The model under review builds one solid part; all positions refer to its coordinate system, in mm. Face numbers are marked on the shaded views. A direction names the side the tool comes from. Coordinates: 2 decimals unless noted, no trailing zeros. Order: outer loops, then holes, each group sorted by start corner. A loop starts at its lowest first (then second) coordinate and runs counter-clockwise, first axis right, second up. Notation, with made-up numbers: M 19.5,-10 L 54.5,-10 A18 ccw 54.5,-2 Z; hole C -4,1.25 d7. An arc over 180 degrees is marked long. Answer in a Markdown table with one row per item.
from build123d import *

# Parameters (mm, degrees)
CHAMFER_1_SIZE      = 1.1015
SKETCH_2_W          = 50
SKETCH_2_H          = 3
CUT_EXTRUDE_1_DEPTH = 3.892099643


with BuildPart() as part:
    # Эскиз1 → Повернуть1 (revolve)
    with BuildSketch(Plane.XY):
        with BuildLine():
            Line((0, 12), (5, 12))
            ThreePointArc((5, 12), (8.36795896, 7.179530606), (9.892099643, 1.5))
            Line((9.892099643, 1.5), (7, 1.5))
            Line((7, 1.5), (7, 0))
            Line((7, 0), (3.5, 0))
            Line((3.5, 0), (3.5, 7.5))
            Line((3.5, 7.5), (0, 7.5))
            Line((0, 7.5), (0, 12))
        make_face()
    revolve(axis=Axis((0, 0, 0), (1, 0, 0)))

    # Фаска1
    chamfer_1_edges = [part.edges().sort_by_distance(p)[0] for p in [
        (0, -12, 0),
    ]]
    chamfer(chamfer_1_edges, length=CHAMFER_1_SIZE)

    # Эскиз2 → Вырез-Вытянуть1 (cut, through all)
    with BuildSketch(Plane(origin=(7, 0, 0), x_dir=(0, 0, -1), z_dir=(1, 0, 0))):
        Rectangle(SKETCH_2_W, SKETCH_2_H)
    extrude(amount=CUT_EXTRUDE_1_DEPTH, mode=Mode.SUBTRACT)


solid = part.part
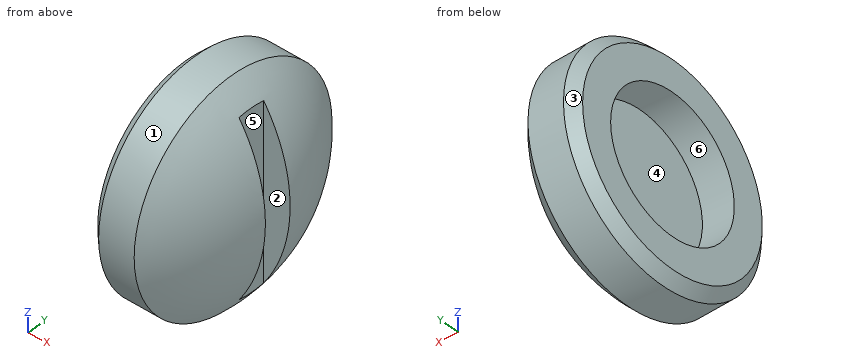
(1) Take a section at A-A (y = 0). Write out the cut boundary in (x, z), then the cut area to 3 significant figures.
Report:
| item | result |
|---|---|
| outline | M 0,-10.9 L 1.1,-12 L 5,-12 A17 ccw 7,-9.58 L 7,9.58 A17 ccw 5,12 L 1.1,12 L 0,10.9 L 0,7.5 L 3.5,7.5 L 3.5,-7.5 L 0,-7.5 Z |
| area | 110 mm^2 |
(2) The part is to be moulded in two halves that separate along Z. For the marked faces 3, 4, 5 and 6, say which applies: +Z half, -Z half, draft (parallel to the pull), parting line (faces both ways), or undercut.
Report:
| item | result |
|---|---|
| face 3 | parting line |
| face 4 | undercut |
| face 5 | draft |
| face 6 | undercut |
(3) Insertion check: P1, Ø3.5, axis at y = 0, z = -3, coming from the +X side; P2, Ø1, axis at x = 4.5, y = -7.5, coming from the -Z side; P3, Ø12, axis at y = 0, z = -0.5, coming from the -X side. Each pin has a flat end and moves straight along its axis. Give the tip position at first contact, or say it passes through.
Report:
| item | result |
|---|---|
| P1 | x = 9.76 |
| P2 | z = -9.75 |
| P3 | x = 3.5 |
(4) Take a section at B-B (x = 2). Write out the cut boundary in (y, z).
Report:
| item | result |
|---|---|
| outline | C 0,0 d24; hole C 0,0 d15 |
(5) Take a section at C-C (x = 5.75). Write out the cut boundary in (y, z), then the cut area to 3 significant figures.
Report:
| item | result |
|---|---|
| outline | C 0,0 d22.39 |
| area | 394 mm^2 |
(6) To check wall thickness, follow line 1 (Z direction, x = 1.55, y = 0); line 2 (Y direction, x = 8.75, z = 0.75); line 3 (X direction, y = 8.75, z = -1). State the ranges of each line that lie inside material, in increasing order. Write a range as [from, to].
Report:
| item | result |
|---|---|
| line 1 | [-12, -7.5], [7.5, 12] |
| line 2 | [-6.25, -1.5], [1.5, 6.25] |
| line 3 | [0, 7.5] |
(7) Machinability: for the marked faces 1 and 2, which of the approach directions +Z, -Z, +X, -X, +Y, -Y give a long, thin tool a straight path to every point of the face, cutting with its end or side? Answer none if there is none.
Report:
| item | result |
|---|---|
| face 1 | +X, -X |
| face 2 | +Z, -Z, +X |
